```python
from build123d import *

# Parameters (mm, degrees)
F0_R     = 0.9
F0_R_2   = 2
F1_DEPTH = 1.5
F2_R     = 2


with BuildPart() as f1:
    # F0 (on Top) → F1 (new body)
    with BuildSketch(Plane.XY):
        with BuildLine():
            ThreePointArc((2.21325, 5.845), (0, 4), (-2.21325, 5.845))
            ThreePointArc((-2.21325, 5.845), (-4.419417, 4.419417), (-5.845, 2.21325))
            ThreePointArc((-5.845, 2.21325), (-4, 0), (-5.845, -2.21325))
            ThreePointArc((-5.845, -2.21325), (-4.419417, -4.419417), (-2.21325, -5.845))
            ThreePointArc((-2.21325, -5.845), (0, -4), (2.21325, -5.845))
            ThreePointArc((2.21325, -5.845), (4.419417, -4.419417), (5.845, -2.21325))
            ThreePointArc((5.845, -2.21325), (4, 0), (5.845, 2.21325))
            ThreePointArc((5.845, 2.21325), (4.419417, 4.419417), (2.21325, 5.845))
        make_face()
        with Locations((-3.181981, -3.181981)):
            Circle(F0_R, mode=Mode.SUBTRACT)
        with Locations((3.181981, -3.181981)):
            Circle(F0_R, mode=Mode.SUBTRACT)
        Circle(F0_R_2, mode=Mode.SUBTRACT)
        with Locations((-3.181981, 3.181981)):
            Circle(F0_R, mode=Mode.SUBTRACT)
        with Locations((3.181981, 3.181981)):
            Circle(F0_R, mode=Mode.SUBTRACT)
    extrude(amount=F1_DEPTH)

    # F2
    f2_edges = [f1.edges().sort_by_distance(p)[0] for p in [
        (2.21325, -5.845, 0.75),
        (-2.21325, -5.845, 0.75),
        (5.845, -2.21325, 0.75),
        (5.845, 2.21325, 0.75),
        (-5.845, -2.21325, 0.75),
        (-2.21325, 5.845, 0.75),
        (2.21325, 5.845, 0.75),
        (-5.845, 2.21325, 0.75),
    ]]
    fillet(f2_edges, radius=F2_R)


solid = f1.part
```
Source: CAD feature listing. Evaluate the final solid. Frame: model axes, mm. Round coordinates to 2 decimals unless told otherwise and drop trailing zeros. Loops run counter-clockwise (first coordinate to the right, second up) from the corner with the lowest first, then second, coordinate; pieces in that order, holes last. Notation, with made-up numbers: M 51,0.5 L 85,0.5 A23 ccw 85,39.5 Z; hole C -6,22 d10. An arc over 180 degrees is marked long. Use a Markdown table: item, result. Add a question column.
1. Cut plane A-A, the plane x = 0. Output: boundary loops of the cut face in (y, z), and give its area (3 significant figures).
2. Ray query, line 1 along X through (y, z) = (2.5, 0.9); line 2 along Y through (x, z) = (-3, 1.35); line 3 along Y through (x, z) = (-3.5, 1.3). Return the intervals inside material, ascending. Write a range as [from, to].
3. Cut plane C-C, the plane x = 2.75. State how many separate pieces and enclosed holes the cut face has, and give its area (3 significant figures).
4. Pull-direction query (X, two-part tool) for faces 1 (the flat face through (-0.1, -2.2, 0)), 2 (the cylindrical face through (0, -2, 1)), 3 (the cylindrical face through (4, 0, 1)); classes: +X half, -X half, draft (parallel to the pull), parting line (faces both ways), or undercut.
Solution:
| question | item | result |
|---|---|---|
| 1 | outline | M -4,0 L -2,0 L -2,1.5 L -4,1.5 Z; M 2,0 L 4,0 L 4,1.5 L 2,1.5 Z |
| 1 | area | 6.00 mm2 |
| 2 | line 1 | x = [-5.09, -3.77], [-2.59, 2.59], [3.77, 5.09] |
| 2 | line 2 | y = [-5.12, -4.06], [-2.3, 2.3], [4.06, 5.12] |
| 2 | line 3 | y = [-5.03, -4.02], [-2.34, 2.34], [4.02, 5.03] |
| 3 | separate pieces | 3 |
| 3 | enclosed holes | 0 |
| 3 | area | 10.6 mm2 |
| 4 | face 1 | draft |
| 4 | face 2 | undercut |
| 4 | face 3 | +X half |
